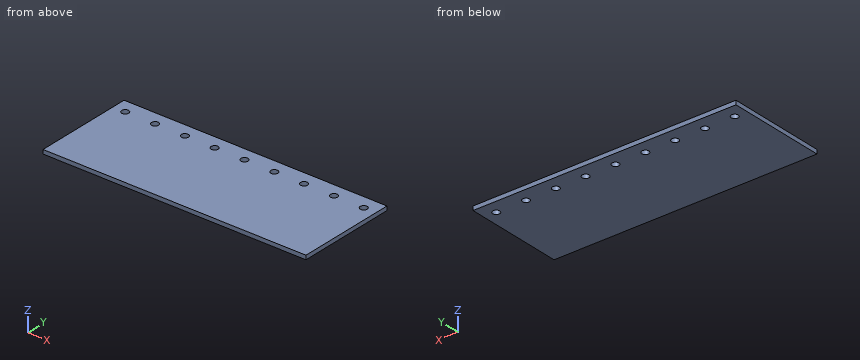
```python
from build123d import *

# Parameters (mm, degrees)
SKETCH_1_W                 = 200
SKETCH_1_H                 = 73.5
EXTRUDE_1_DEPTH            = 3
SKETCH_2_R                 = 2.6
CUT_EXTRUDE_2_DEPTH        = 107.581248351
PATTERN_LINEAR_1_COUNT     = 5
PATTERN_LINEAR_1_PITCH     = 22
PATTERN_LINEAR_1_COL_COUNT = 5
PATTERN_LINEAR_1_COL_PITCH = 22
CUT_EXTRUDE_3_DEPTH        = 107.581248351
CUT_EXTRUDE_3_DEPTH_BACK   = 107.581248351
SKETCH_3_W                 = 3
SKETCH_3_H                 = 73.5


with BuildPart() as part:
    # 草图1 → 凸台-拉伸1 (new body)
    with BuildSketch(Plane.XY):
        Rectangle(SKETCH_1_W, SKETCH_1_H)
    extrude(amount=EXTRUDE_1_DEPTH)

    # 草图2 → 切除-拉伸2 (cut, symmetric)
    with BuildSketch(Plane.XY.offset(3)):
        with Locations((0, 26.75)):
            Circle(SKETCH_2_R)
    cut_extrude_2 = extrude(amount=CUT_EXTRUDE_2_DEPTH, both=True, mode=Mode.SUBTRACT)

    # 阵列(线性)1: 切除-拉伸2 ×5
    with Locations(*[(i * PATTERN_LINEAR_1_PITCH, 0, 0) for i in range(1, PATTERN_LINEAR_1_COUNT)]):
        add(cut_extrude_2, mode=Mode.SUBTRACT)

    # 阵列(线性)1 col: 切除-拉伸2 ×5
    with Locations(*[(-i * PATTERN_LINEAR_1_COL_PITCH, 0, 0) for i in range(1, PATTERN_LINEAR_1_COL_COUNT)]):
        add(cut_extrude_2, mode=Mode.SUBTRACT)

    # 草图3 → 切除-拉伸3 (cut, two sides: drawn at the far end of the back side and taken through both)
    with BuildSketch(Plane.XY.offset(3).offset(-CUT_EXTRUDE_3_DEPTH_BACK)):
        with Locations((-98.5, 0)):
            Rectangle(SKETCH_3_W, SKETCH_3_H)
        with Locations((98.5, 0)):
            Rectangle(SKETCH_3_W, SKETCH_3_H)
    extrude(amount=CUT_EXTRUDE_3_DEPTH + CUT_EXTRUDE_3_DEPTH_BACK, mode=Mode.SUBTRACT)


solid = part.part
```
Part model, mm, in its own coordinate system. Coordinates: 2 decimals unless noted, no trailing zeros. Order: outer loops, then holes, each group sorted by start corner. A loop starts at its lowest first (then second) coordinate and runs counter-clockwise, first axis right, second up. Notation, with made-up numbers: (71, -27.5) - (79, -27.5) arc R13 ccw to (79, -7.5) - close; hole circle Ø9 at (64.5, 49.5). An arc over 180 degrees is marked (long way). Return JSON: item names as keys, results as strings. Group by question number.
Item 1: Cut at B-B (y = 26.75). State how many separate pieces and enclosed holes the cut face has, plus the area to 3 significant figures.
Item 2: Cut at A-A (x = 44). List the corners of the cut face in (y, z).
Item 3: Drill centre lines: probe 1 along Y at (x, z) = (44, 1.55); probe 2 along Y at (x, z) = (-23.5, 0.8). Where is each one in solid material? Low to high. Write a range as from..to.
Check values:
{
 "1": {"separate pieces": "10", "enclosed holes": "0", "area": "442 mm2"},
 "2": {"outline": "(-36.75, 0) - (24.15, 0) - (24.15, 3) - (-36.75, 3) - close; (29.35, 0) - (36.75, 0) - (36.75, 3) - (29.35, 3) - close"},
 "3": {"probe 1": "y = -36.75..24.15, 29.35..36.75", "probe 2": "y = -36.75..24.63, 28.87..36.75"}
}
